Model file for the job. Use its own axes, mm. Round coordinates to 2 decimals unless told otherwise and drop trailing zeros. Loops run counter-clockwise (first coordinate to the right, second up) from the corner with the lowest first, then second, coordinate; pieces in that order, holes last. Notation, with made-up numbers: M 41.25,-16.75 L 93.25,-16.75 A34 cw 93.25,16.25 Z; hole C -26,29 d10. An arc over 180 degrees is marked long. Answer in a Markdown table with one row per item.
from build123d import *

# Parameters (mm, degrees)
SKETCH_1_W      = 10
SKETCH_1_H      = 10
EXTRUDE_1_DEPTH = 10
HOLE_WIZARD_1_D = 3.3
HOLE_WIZARD_2_D = 3.3
HOLE_WIZARD_3_D = 3.3


with BuildPart() as part:
    # 草图1 → 凸台-拉伸1 (new body)
    with BuildSketch(Plane(origin=(0, 0, 0), x_dir=(1, 0, 0), z_dir=(0, 1, 0))):
        Rectangle(SKETCH_1_W, SKETCH_1_H)
    extrude(amount=EXTRUDE_1_DEPTH)

    # 孔1 (through all)
    with Locations(Plane(origin=(0, 10, 0), x_dir=(1, 0, 0), z_dir=(0, 1, 0))):
        with Locations((0, 0)):
            Hole(HOLE_WIZARD_1_D / 2)

    # 孔2 (through all)
    with Locations(Plane(origin=(5, 0, 0), x_dir=(0, 0, -1), z_dir=(1, 0, 0))):
        with Locations((0, 5)):
            Hole(HOLE_WIZARD_2_D / 2)

    # 孔3 (through all)
    with Locations(Plane.XY.offset(5)):
        with Locations((0, 5)):
            Hole(HOLE_WIZARD_3_D / 2)


solid = part.part
1. Mould opens along Z. For faces 1 (the flat face through (-5, 3, 0)), 2 (the flat face through (0, 3, 5)), 3 (the flat face through (0, 3, -5)), 4 (the cylindrical face through (-3.11, 6.115, -1.216)) say: +Z half, -Z half, draft (parallel to the pull), parting line (faces both ways), or undercut.
Verdict:
| item | result |
|---|---|
| face 1 | draft |
| face 2 | +Z half |
| face 3 | -Z half |
| face 4 | undercut |
2. Saw through at B-B (y = 6.5). Write the cut outline in (x, z).
Verdict:
| item | result |
|---|---|
| outline | M -5,-5 L -0.69,-5 L -0.69,-1.5 A1.65 cw -1.5,-0.69 L -5,-0.69 Z; M -5,0.69 L -1.5,0.69 A1.65 cw -0.69,1.5 L -0.69,5 L -5,5 Z; M 0.69,-5 L 5,-5 L 5,-0.69 L 1.5,-0.69 A1.65 cw 0.69,-1.5 Z; M 0.69,1.5 A1.65 cw 1.5,0.69 L 5,0.69 L 5,5 L 0.69,5 Z |
3. Saw through at D-D (z = 2). Write the cut outline in (x, y).
Verdict:
| item | result |
|---|---|
| outline | M -5,0 L 5,0 L 5,10 L -5,10 Z; hole C 0,5 d3.3 |
4. Saw through at C-C (x = -0.5). Write the cut outline in (y, z), and give its area (3 significant figures).
Verdict:
| item | result |
|---|---|
| outline | M 0,-5 L 3.43,-5 L 3.43,-1.57 L 0,-1.57 Z; M 0,1.57 L 3.43,1.57 L 3.43,5 L 0,5 Z; M 6.57,-5 L 10,-5 L 10,-1.57 L 6.57,-1.57 Z; M 6.57,1.57 L 10,1.57 L 10,5 L 6.57,5 Z |
| area | 47.0 mm² |
5. Wall check: probe 1 along X at (y, z) = (5, 2.95); probe 2 along Y at (x, z) = (0, 1.9). Give the ranges that are in metal, low to high.
Verdict:
| item | result |
|---|---|
| probe 1 | x = -5 to -1.65, 1.65 to 5 |
| probe 2 | y = 0 to 3.35, 6.65 to 10 |
6. Saw through at A-A (z = 0). Write the cut outline in (x, y), and give its area (3 significant figures).
Verdict:
| item | result |
|---|---|
| outline | M -5,0 L -1.65,0 L -1.65,3.35 L -5,3.35 Z; M -5,6.65 L -1.65,6.65 L -1.65,10 L -5,10 Z; M 1.65,0 L 5,0 L 5,3.35 L 1.65,3.35 Z; M 1.65,6.65 L 5,6.65 L 5,10 L 1.65,10 Z |
| area | 44.9 mm² |
